Source: CAD feature listing. Evaluate the final solid. Frame: model axes, mm. Face numbers are marked on the shaded views. A direction names the side the tool comes from. Give positions to 0.01 mm unless a question says otherwise; leave off trailing zeros. Order: outer loops, then holes, each group sorted by start corner. A loop starts at its lowest first (then second) coordinate and runs counter-clockwise, first axis right, second up. Notation, with made-up numbers: M 28,60 L 45,60 A26 cw 45,93 Z; hole C -35.5,53 d2. An arc over 180 degrees is marked long. Return JSON: item names as keys, results as strings.
from build123d import *

# Parameters (mm, degrees)
SKETCH1_W           = 11
SKETCH1_H           = 22
BOSS_EXTRUDE1_DEPTH = 2
SKETCH2_R           = 3
BOSS_EXTRUDE2_DEPTH = 4
FILLET1_R           = 0.5


with BuildPart() as part:
    # Sketch1 → Boss-Extrude1 (new body)
    with BuildSketch(Plane.XY):
        with Locations((-6, 0)):
            Rectangle(SKETCH1_W, SKETCH1_H)
    extrude(amount=BOSS_EXTRUDE1_DEPTH)

    # Sketch2 → Boss-Extrude2 (add)
    with BuildSketch(Plane.XY.offset(2)):
        with Locations(Location((-6, 5.25, 0), (0, 0, 180))):
            Circle(SKETCH2_R)
    extrude(amount=BOSS_EXTRUDE2_DEPTH)

    # Fillet1
    fillet1_edges = [part.edges().sort_by_distance(p)[0] for p in [
        (-3, 5.25, 6),
        (-11.5, 11, 1),
        (-0.5, 11, 1),
        (-0.5, -11, 1),
        (-11.5, -11, 1),
    ]]
    fillet(fillet1_edges, radius=FILLET1_R)


solid = part.part
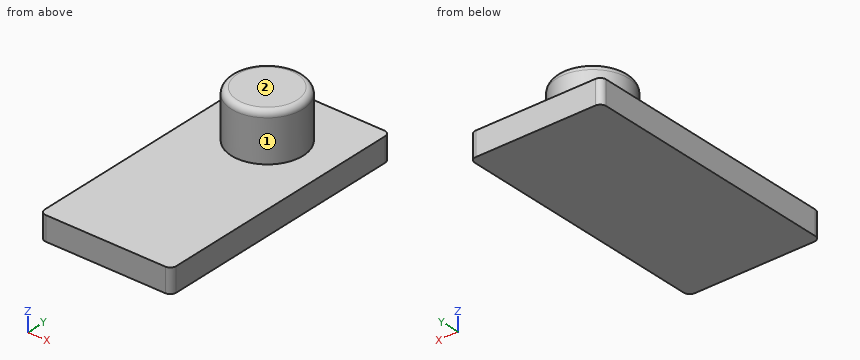
1. Set-up query: the marked faces 1 and 2. Return all of +Z, -Z, +X, -X, +Y, -Y with unobstructed straight access to the full face (end or side cutting, diameter ignored); none if empty.
Evaluation:
{"face 1": "+Z", "face 2": "+Z, +X, -X, +Y, -Y"}
2. Ray query, probe 1 along Z at (x, y) = (-1.5, 3); probe 2 along X at (y, z) = (5.25, 3.45); probe 3 along X at (y, z) = (7.75, 3.9). Return the intervals inside material, ascending.
Evaluation:
{"probe 1": "z = 0 to 2", "probe 2": "x = -9 to -3", "probe 3": "x = -7.66 to -4.34"}
3. Section query B-B (y = 5.25). Return loops of the section in (x, z).
Evaluation:
{"outline": "M -11.5,0 L -0.5,0 L -0.5,2 L -3,2 L -3,5.5 A0.5 ccw -3.5,6 L -8.5,6 A0.5 ccw -9,5.5 L -9,2 L -11.5,2 Z"}
4. First-contact query: pin 1 (1.5 mm diameter, centred on y = 3, z = 2.5, fed in from -X); pin 2 (3 mm diameter, centred on x = -10, z = 4.5, fed in from +Y); pin 3 (2 mm diameter, centred on x = -9.5, y = 2.5, fed in from +Z); pin 4 (1.5 mm diameter, centred on y = 4.5, z = 3, fed in from -X). Flat tips, straight axial feed; report the tip coordinate or a pass-through.
Evaluation:
{"pin 1": "stops at x = -11.5", "pin 2": "stops at y = 6.91", "pin 3": "stops at z = 2", "pin 4": "stops at x = -9"}
5. Section query A-A (x = -6). Return loops of the section in (y, z), then the cut area to 3 significant figures.
Evaluation:
{"outline": "M -11,0 L 11,0 L 11,2 L 8.25,2 L 8.25,5.5 A0.5 ccw 7.75,6 L 2.75,6 A0.5 ccw 2.25,5.5 L 2.25,2 L -11,2 Z", "area": "67.9 mm^2"}
6. Section query C-C (z = 3.1). Return loops of the section in (x, y).
Evaluation:
{"outline": "C -6,5.25 d6"}
7. Section query D-D (y = -1.75). Return loops of the section in (x, z), then the cut area to 3 significant figures.
Evaluation:
{"outline": "M -11.5,0 L -0.5,0 L -0.5,2 L -11.5,2 Z", "area": "22.0 mm^2"}
